Check sheet for the drawn part. Datum: minimum x, y, z corner. Units: mm. Give positions to 0.01 mm unless a question says otherwise; leave off trailing zeros. Write item = value, one per line. Start each with the question number.
1. Thickness scan on line 1 along X through (y, z) = (25, 1.1); line 2 along X through (y, z) = (127, 0.75); line 3 along Y through (x, z) = (73.5, 0.5). Record the ranges inside material, lowest first.
2. Depth check by flat-ended pin: P1, Ø1, axis at y = 182.5, z = 1, coming from the +X side; P2, Ø1, axis at y = 70.5, z = 0.5, coming from the -X side. Enter the tip coordinate at first touch or a pass-through.
3. Cross-section at A-A, the plane z = 1.55. State how many separate pieces and enclosed holes the cut face has, plus the area to 3 significant figures.
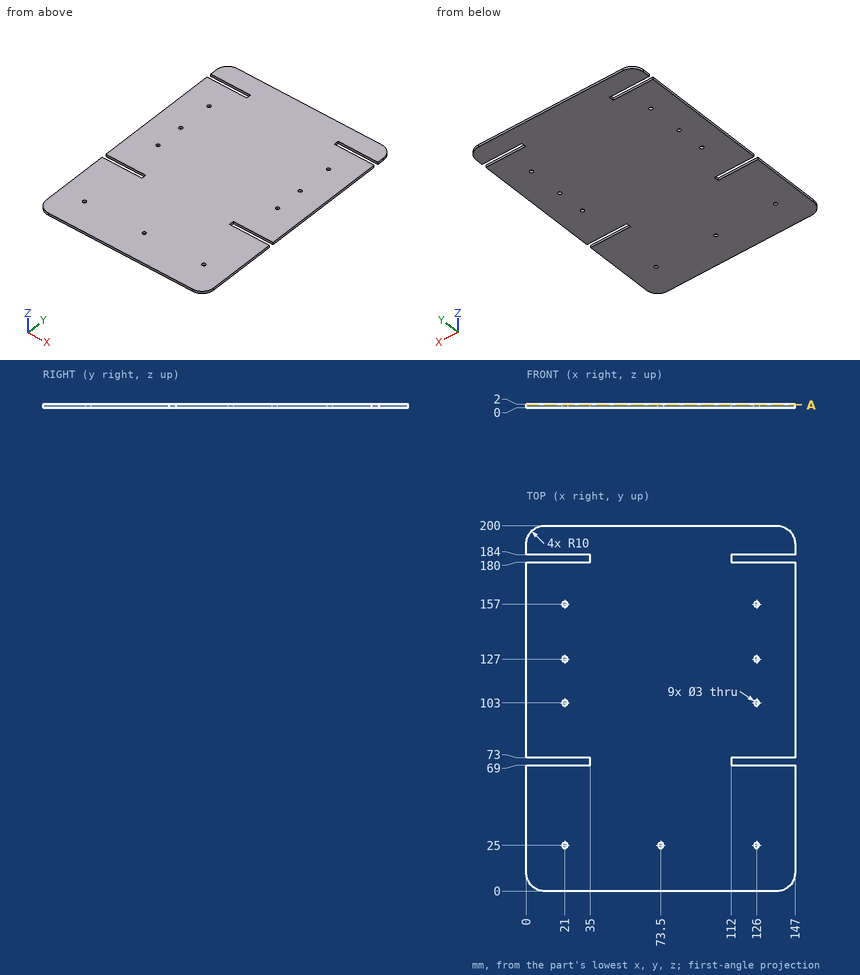
Answers:
q1.line_1 = 0 to 19.5, 22.5 to 72, 75 to 124.5, 127.5 to 147
q1.line_2 = 0 to 19.5, 22.5 to 124.5, 127.5 to 147
q1.line_3 = 0 to 23.5, 26.5 to 200
q2.P1 = 112
q2.P2 = 35
q3.separate_pieces = 1
q3.enclosed_holes = 9
q3.area = 28,700 mm^2
